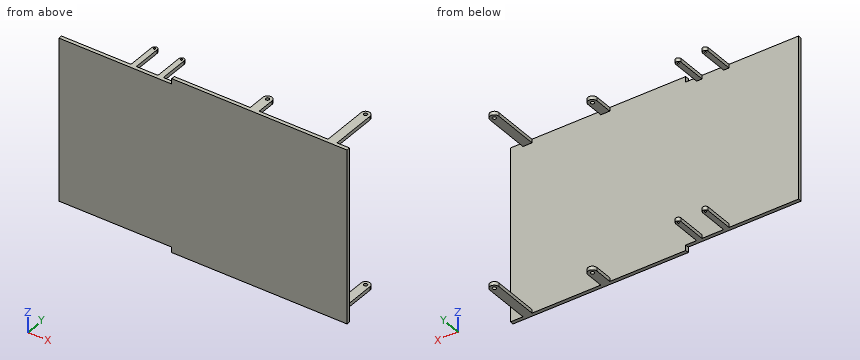
```python
from build123d import *

# Parameters (mm, degrees)
BOSS_EXTRUDE1_DEPTH = 20
SKETCH2_R           = 10
BOSS_EXTRUDE2_DEPTH = 20
SKETCH3_R           = 5
BOSS_EXTRUDE3_DEPTH = 20


with BuildPart() as part:
    # Sketch1 → Boss-Extrude1 (new body)
    with BuildSketch(Plane(origin=(0, 0, 0), x_dir=(1, 0, 0), z_dir=(0, 1, 0))):
        Polygon((-173.422280891, 480), (-173.422280891, 450), (-800, 450), (-800, -450), (-173.422280891, -450), (-173.422280891, -480), (800, -480), (800, 480), align=None)
    extrude(amount=-BOSS_EXTRUDE1_DEPTH)

    # Sketch2 → Boss-Extrude2 (add)
    with BuildSketch(Plane.XY.offset(480)):
        with BuildLine():
            Line((248, 0), (298, 0))
            Line((298, 0), (298, 100))
            ThreePointArc((298, 100), (273, 125), (248, 100))
            Line((248, 100), (248, 0))
        make_face()
        with Locations((273, 100)):
            Circle(SKETCH2_R, mode=Mode.SUBTRACT)
        with BuildLine():
            Line((680, 258.2), (680, 0))
            Line((680, 0), (730, 0))
            Line((730, 0), (730, 258.2))
            ThreePointArc((730, 258.2), (705, 283.2), (680, 258.2))
        make_face()
        with Locations((705, 258.2)):
            Circle(SKETCH2_R, mode=Mode.SUBTRACT)
        Polygon((680, 0), (298, 0), (248, 0), (-173.422280891, 0), (-173.422280891, -20), (800, -20), (800, 0), (730, 0), align=None)
    extrude(amount=-BOSS_EXTRUDE2_DEPTH)

    # Mirror1: part across plane


with BuildPart() as part_1:
    add(part.part)
    add(part.part.mirror(Plane.XY))

    # Sketch3 → Boss-Extrude3 (add)
    with BuildSketch(Plane.XY.offset(450)):
        with BuildLine():
            Line((-414, 0), (-384, 0))
            Line((-384, 0), (-384, 162.7))
            ThreePointArc((-384, 162.7), (-399, 177.7), (-414, 162.7))
            Line((-414, 162.7), (-414, 0))
        make_face()
        with Locations((-399, 162.7)):
            Circle(SKETCH3_R, mode=Mode.SUBTRACT)
        with BuildLine():
            Line((-264, 0), (-234, 0))
            Line((-234, 0), (-234, 162.7))
            ThreePointArc((-234, 162.7), (-249, 177.7), (-264, 162.7))
            Line((-264, 162.7), (-264, 0))
        make_face()
        with Locations((-249, 162.7)):
            Circle(SKETCH3_R, mode=Mode.SUBTRACT)
    boss_extrude3 = extrude(amount=-BOSS_EXTRUDE3_DEPTH)

    # Mirror2: Boss-Extrude3 across plane
    add(boss_extrude3.mirror(Plane.XY))


solid = part_1.part
```
The listing builds one solid part. Answer for the finished solid, in the listing's coordinates (mm). Coordinates: 2 decimals unless noted, no trailing zeros. Write each loop counter-clockwise with the first axis right and the second up, starting at its lowest first coordinate (ties: lowest second). Pieces come first, ordered by that corner, then holes. Notation, with made-up numbers: (-3, 42.25) - (44, 42.25) arc R28 cw to (44, 61.25) - close; hole circle Ø10 at (-5, 68). An arc over 180 degrees is marked (long way). Return JSON: item names as keys, results as strings. Group by question number.
Q1. Find the intervals of material crossed by line 1 along X through (y, z) = (162, -434); line 2 along Y through (x, z) = (705, -467); line 3 along Y through (x, z) = (651, 374.5), in increasing order. Write a range as [from, to].
Q2. The part is cut by section B-B on z = -135. Write down the section's boundary in (x, y), and give its area (3 significant figures).
Q3. Flat-ended cylindrical pins translate along their axes: pin 1 Ø10 at (y, z) = (50.5, 474) entering from +X; pin 2 Ø10 at (y, z) = (32, -471.5) entering from -X; pin 3 Ø3 at (x, z) = (7.5, 14) entering from +Y. Find the tip coordinate at first contact, or state that the pin passes through.
Q4. The part is cut by section A-A on y = 45. State how many separate pieces and enclosed holes the cut face has, and give its area (3 significant figures).
Q5. The part is cut by section C-C on x = -696. Write down the section's boundary in (y, z), and give its area (3 significant figures).
Evaluation:
{
 "1": {"line 1": "x = [-414, -403.95], [-394.05, -384], [-264, -253.95], [-244.05, -234]", "line 2": "y = [-20, 248.2], [268.2, 283.2]", "line 3": "y = [-20, 0]"},
 "2": {"outline": "(-800, -20) - (800, -20) - (800, 0) - (-800, 0) - close", "area": "32,000 mm2"},
 "3": {"pin 1": "stops at x = 730", "pin 2": "stops at x = 248", "pin 3": "stops at y = 0"},
 "4": {"separate pieces": "8", "enclosed holes": "0", "area": "6,400 mm2"},
 "5": {"outline": "(-20, -450) - (0, -450) - (0, 450) - (-20, 450) - close", "area": "18,000 mm2"}
}
